Model file for the job. Use its own axes, mm. Face numbers are marked on the shaded views. A direction names the side the tool comes from. Round coordinates to 2 decimals unless told otherwise and drop trailing zeros. Loops run counter-clockwise (first coordinate to the right, second up) from the corner with the lowest first, then second, coordinate; pieces in that order, holes last. Notation, with made-up numbers: M 3,42 L 22,42 A27 cw 22,68 Z; hole C 74,85 d6. An arc over 180 degrees is marked long. Answer in a Markdown table with one row per item.
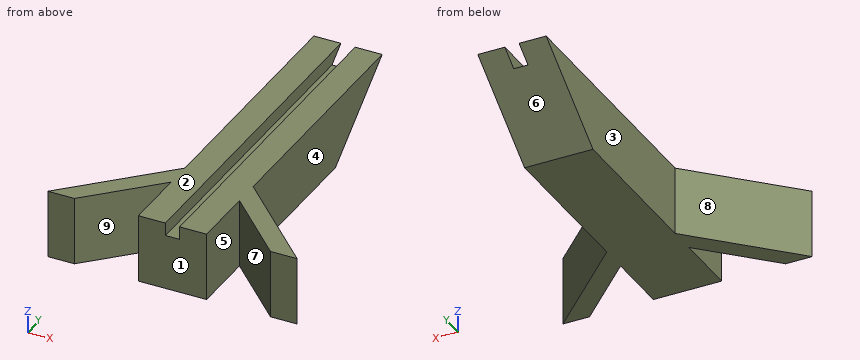
from build123d import *

# Parameters (mm, degrees)
SKETCH1_W           = 30
SKETCH1_H           = 30
BOSS_EXTRUDE1_DEPTH = 150
BOSS_EXTRUDE2_DEPTH = 15
CUT_EXTRUDE1_DEPTH  = 70.736433232
SKETCH4_W           = 6.25
SKETCH4_H           = 11.445552978
CUT_EXTRUDE2_DEPTH  = 151


with BuildPart() as part:
    # Sketch1 → Boss-Extrude1 (new body)
    with BuildSketch(Plane(origin=(0, 0, 0), x_dir=(1, 0, 0), z_dir=(0, 1, 0))):
        Rectangle(SKETCH1_W, SKETCH1_H)
    extrude(amount=BOSS_EXTRUDE1_DEPTH)

    # Sketch2 → Boss-Extrude2 (add, symmetric)
    with BuildSketch(Plane.XY):
        Polygon((15, 39.736433232), (54.736433232, 0), (43.033817395, 0), (15, 28.033817395), align=None)
    boss_extrude2 = extrude(amount=BOSS_EXTRUDE2_DEPTH, both=True)

    # Mirror1: Boss-Extrude2 across plane
    add(boss_extrude2.mirror(Plane(origin=(0, 0, 0), x_dir=(0, 0, 1), z_dir=(1, 0, 0))))

    # Sketch3 → Cut-Extrude1 (cut, through all)
    with BuildSketch(Plane.ZY.offset(15)):
        Polygon((15, 150), (-15, 110), (-15, 150), align=None)
    extrude(amount=-CUT_EXTRUDE1_DEPTH, mode=Mode.SUBTRACT)

    # Sketch4 → Cut-Extrude2 (cut, through all)
    with BuildSketch(Plane.XZ):
        with Locations((0, 15)):
            Rectangle(SKETCH4_W, SKETCH4_H)
    extrude(amount=-CUT_EXTRUDE2_DEPTH, mode=Mode.SUBTRACT)


solid = part.part
1. Pin check, flat tips, straight feed: pin 1 (5 mm diameter, centred on y = 98, z = 0, fed in from +X); pin 2 (1 mm diameter, centred on y = 21.5, z = 9.5, fed in from -X); pin 3 (3 mm diameter, centred on x = 1.5, y = 57.5, fed in from +Z). Stop position of each tip, or through.
Verdict:
| item | result |
|---|---|
| pin 1 | stops at x = 15 |
| pin 2 | stops at x = -33.74 |
| pin 3 | stops at z = 9.28 |
2. Saw through at A-A (z = 0). Write the cut outline in (x, y), and give its area (3 significant figures).
Verdict:
| item | result |
|---|---|
| outline | M -54.74,0 L -43.03,0 L -15,28.03 L -15,0 L 15,0 L 15,28.03 L 43.03,0 L 54.74,0 L 15,39.74 L 15,130 L -15,130 L -15,39.74 Z |
| area | 4,690 mm² |
3. Saw through at D-D (z = 13.25). Write the cut outline in (x, y) (3 decimals).
Verdict:
| item | result |
|---|---|
| outline | M -54.736,0 L -43.034,0 L -15,28.034 L -15,0 L -3.125,0 L -3.125,147.667 L -15,147.667 L -15,39.736 Z; M 3.125,0 L 15,0 L 15,28.034 L 43.034,0 L 54.736,0 L 15,39.736 L 15,147.667 L 3.125,147.667 Z |
4. Tool access for the marked faces 1, 2, 3, 4 and 5: list every direction of +Z, -Z, +X, -X, +Y, -Y with a clear straight run to the whole face (end or side of a thin tool).
Verdict:
| item | result |
|---|---|
| face 1 | +Z, -Z, +X, -X, -Y |
| face 2 | +Z, +X, -X, +Y, -Y |
| face 3 | +Z, -Z, -X, +Y |
| face 4 | +Z, -Z, +X, +Y |
| face 5 | +Z, -Z, -Y |
5. Wall check: probe 1 along X at (y, z) = (27.5, -8); probe 2 along X at (y, z) = (51, -5.5); probe 3 along X at (y, z) = (24.5, 1.75). Give the ranges that are in metal, low to high.
Verdict:
| item | result |
|---|---|
| probe 1 | x = -27.24 to -15.53, -15 to 15, 15.53 to 27.24 |
| probe 2 | x = -15 to 15 |
| probe 3 | x = -30.24 to -18.53, -15 to 15, 18.53 to 30.24 |
6. Saw through at B-B (y = 10.5). Write the cut outline in (x, z) (3 decimals), and give its area (3 significant figures).
Verdict:
| item | result |
|---|---|
| outline | M -44.236,-15 L -32.534,-15 L -32.534,15 L -44.236,15 Z; M -15,-15 L 15,-15 L 15,15 L 3.125,15 L 3.125,9.277 L -3.125,9.277 L -3.125,15 L -15,15 Z; M 32.534,-15 L 44.236,-15 L 44.236,15 L 32.534,15 Z |
| area | 1,570 mm² |
7. Mould opens along X. For the marked faces 6, 7, 8 and 9 say: +X half, -X half, draft (parallel to the pull), parting line (faces both ways), or undercut.
Verdict:
| item | result |
|---|---|
| face 6 | draft |
| face 7 | undercut |
| face 8 | -X half |
| face 9 | undercut |
8. Saw through at C-C (y = 134). Write the cut outline in (x, z) (3 decimals).
Verdict:
| item | result |
|---|---|
| outline | M -15,3 L 15,3 L 15,15 L 3.125,15 L 3.125,9.277 L -3.125,9.277 L -3.125,15 L -15,15 Z |
